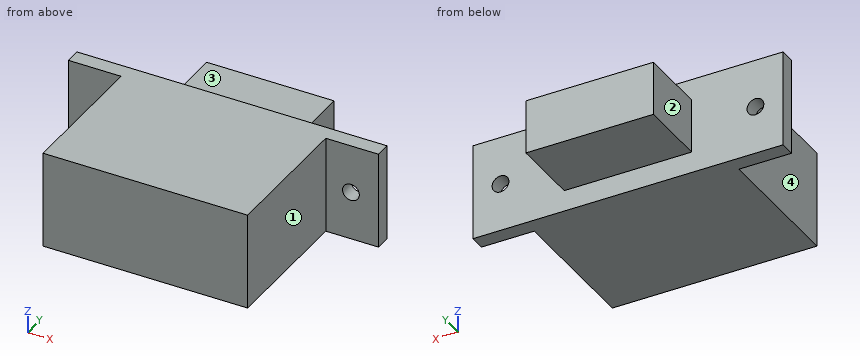
Autodesk Inventor part; units mm, degrees
ref_plane "XZ Plane" through (0, 0, 0) normal (0, 1, 0) x (-1, 0, 0)
ref_plane "XY Plane" through (0, 0, 0) normal (0, 0, 1) x (1, 0, 0)
sketch "Sketch1" plane through (0, 0, 0) normal (0, 1, 0) x (-1, 0, 0)
  line L0 (-11.55, 3.6125) -> (11.55, 3.6125)
  line L1 (11.55, 3.6125) -> (11.55, -3.6125)
  line L2 (11.55, -3.6125) -> (-11.55, -3.6125)
  line L3 (-11.55, -3.6125) -> (-11.55, 3.6125)
  line L4 (-11.55, 3.6125) -> (11.55, -3.6125) construction
  line L5 (11.55, 3.6125) -> (-11.55, -3.6125) construction
  point P0 (0, 0)
  dimension "d0" = 23.1
  dimension "d1" = 7.225
extrude "Extrusion1" add sketch "Sketch1" along normal blind 1.15
sketch "Sketch2" plane through (0, 0, 0) normal (0, -1, 0) x (1, 0, 0)
  line L0 (-11.55, 3.6125) -> (11.55, 3.6125)
  line L1 (-7.625, -3.6125) -> (7.625, -3.6125)
  line L2 (7.625, -3.6125) -> (7.625, 3.6125)
  line L3 (7.625, 3.6125) -> (-7.625, 3.6125)
  line L4 (-7.625, 3.6125) -> (-7.625, -3.6125)
  line L5 (-7.625, -3.6125) -> (7.625, 3.6125) construction
  line L6 (7.625, -3.6125) -> (-7.625, 3.6125) construction
  point P0 (0, 0)
  dimension "d4" = 15.25
extrude "Extrusion2" add sketch "Sketch2" along normal blind 10.5
sketch "Sketch3" plane through (0, 1.15, 0) normal (0, 1, 0) x (1, 0, 0)
  line L0 (-4.75, -2.025) -> (4.75, -2.025)
  line L1 (4.75, -2.025) -> (4.75, 2.025)
  line L2 (4.75, 2.025) -> (-4.75, 2.025)
  line L3 (-4.75, 2.025) -> (-4.75, -2.025)
  line L4 (-4.75, -2.025) -> (4.75, 2.025) construction
  line L5 (4.75, -2.025) -> (-4.75, 2.025) construction
  point P0 (0, 0)
  dimension "d7" = 9.5
  dimension "d8" = 4.05
extrude "Extrusion3" add sketch "Sketch3" along normal blind 5.15
sketch "Sketch4" plane through (0, 1.15, 0) normal (0, 1, 0) x (1, 0, 0)
  line L0 (11.55, 3.6125) -> (-11.55, 3.6125) construction
  line L1 (0, 3.6125) -> (0, -3.6125) construction
  line L2 (-11.55, -3.6125) -> (11.55, -3.6125) construction
  line L3 (-11.55, 3.6125) -> (-11.55, -3.6125) construction
  line L4 (-11.55, 0) -> (11.55, 0) construction
  line L5 (11.55, -3.6125) -> (11.55, 3.6125) construction
  circle A0 centre (9.5, 0) radius 0.625
  circle A1 centre (-9.5, 0) radius 0.625
  point P0 (0, 0)
  dimension "d11" = 1.25
  dimension "d12" = 9.5
extrude "Extrusion4" cut sketch "Sketch4" against normal up to surface (1.15 mm away)
properties part number "Switch"
Verification items for the finished model (mm, model axes). Face numbers are marked on the shaded views. A direction names the side the tool comes from. Round coordinates to 2 decimals unless told otherwise and drop trailing zeros. Write each loop counter-clockwise with the first axis right and the second up, starting at its lowest first coordinate (ties: lowest second). Pieces come first, ordered by that corner, then holes. Notation, with made-up numbers: (-6, 80.5) - (50, 80.5) arc R34 ccw to (50, 111.5) - close; hole circle Ø10 at (37.5, -26.75). An arc over 180 degrees is marked (long way). Answer as a JSON object with one key per item and string values. Group by question number.
Q1. Thickness scan on line 1 (X direction, y = 0.65, z = 0) (3 decimals); line 2 (Z direction, x = -9.5, y = 0.55) (1 decimal); line 3 (X direction, y = 0.5, z = 0.5) (3 decimals). Record the ranges inside material, lowest first.
Q2. Go/stop test with flat-tipped pins: pin 1 Ø2 at (y, z) = (2.5, 0.5) entering from -X; pin 2 Ø1.2 at (x, z) = (10.5, 0.5) entering from -Y; pin 3 Ø1 at (y, z) = (-3.5, -0.5) entering from -X (3 decimals). Record where each tip stops, or that it passes through.
Q3. Section check C-C, the plane z = -3. Enter the section's corners in (x, y) (3 decimals), plus the area to 3 significant figures.
Q4. Section check A-A, the plane z = 0. Enter the section's corners in (x, y) (3 decimals), plus the area to 3 significant figures.
Q5. Tool access check on the marked faces 1, 2, 3 and 4. Record the directions out of +Z, -Z, +X, -X, +Y, -Y that give a thin tool (end or side, any length) a straight path to the whole face; none if there is none.
Found:
{
 "1": {"line 1": "x = -11.55 to -10.125, -8.875 to 8.875, 10.125 to 11.55", "line 2": "z = -3.6 to -0.6, 0.6 to 3.6", "line 3": "x = -11.55 to -9.875, -9.125 to 9.125, 9.875 to 11.55"},
 "2": {"pin 1": "stops at x = -4.75", "pin 2": "stops at y = 0", "pin 3": "stops at x = -7.625"},
 "3": {"outline": "(-11.55, 0) - (-7.625, 0) - (-7.625, -10.5) - (7.625, -10.5) - (7.625, 0) - (11.55, 0) - (11.55, 1.15) - (-11.55, 1.15) - close", "area": "187 mm^2"},
 "4": {"outline": "(-11.55, 0) - (-10.125, 0) - (-10.125, 1.15) - (-11.55, 1.15) - close; (-8.875, 0) - (-7.625, 0) - (-7.625, -10.5) - (7.625, -10.5) - (7.625, 0) - (8.875, 0) - (8.875, 1.15) - (4.75, 1.15) - (4.75, 6.3) - (-4.75, 6.3) - (-4.75, 1.15) - (-8.875, 1.15) - close; (10.125, 0) - (11.55, 0) - (11.55, 1.15) - (10.125, 1.15) - close", "area": "233 mm^2"},
 "5": {"face 1": "+Z, -Z, +X, -Y", "face 2": "+Z, -Z, -X, +Y", "face 3": "+Z, +X, -X, +Y", "face 4": "+Z, -Z, -X, -Y"}
}
